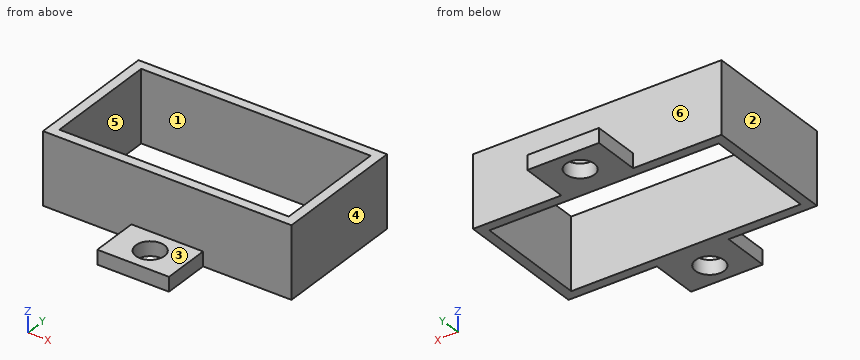
from build123d import *

# Parameters (mm, degrees)
SKETCH_1_W          = 52
SKETCH_1_H          = 28
SKETCH_1_W_2        = 48
SKETCH_1_H_2        = 24
EXTRUDE_1_DEPTH     = 15
SKETCH_2_W          = 15
SKETCH_2_H          = 3
EXTRUDE_2_DEPTH     = 10
SKETCH_3_R          = 3
CUT_EXTRUDE_1_DEPTH = 10


with BuildPart() as part:
    # 草圖1 → 填料-伸長1 (new body)
    with BuildSketch(Plane.XY):
        Rectangle(SKETCH_1_W, SKETCH_1_H)
        Rectangle(SKETCH_1_W_2, SKETCH_1_H_2, mode=Mode.SUBTRACT)
    extrude(amount=EXTRUDE_1_DEPTH)

    # 草圖2 → 填料-伸長2 (add)
    with BuildSketch(Plane(origin=(0, 14, 0), x_dir=(1, 0, 0), z_dir=(0, 1, 0))):
        with Locations((0, -1.5)):
            Rectangle(SKETCH_2_W, SKETCH_2_H)
    extrude_2 = extrude(amount=EXTRUDE_2_DEPTH)

    # 草圖3 → 除料-伸長1 (cut)
    with BuildSketch(Plane.XY.offset(3)):
        with Locations((0, 19)):
            Circle(SKETCH_3_R)
    cut_extrude_1 = extrude(amount=-CUT_EXTRUDE_1_DEPTH, mode=Mode.SUBTRACT)

    # 鏡射1: 填料-伸長2, 除料-伸長1 across plane
    add(extrude_2.mirror(Plane.ZX))
    add(cut_extrude_1.mirror(Plane.ZX), mode=Mode.SUBTRACT)


solid = part.part
Input: part model. Units: mm. Frame: model coordinates. Face numbers are marked on the shaded views. A direction names the side the tool comes from. Coordinates: 2 decimals unless noted, no trailing zeros. Loops run counter-clockwise (first coordinate to the right, second up) from the corner with the lowest first, then second, coordinate; pieces in that order, holes last. Notation, with made-up numbers: (14.5, 2.25) - (25.5, 2.25) arc R20 cw to (25.5, 39.25) - close; hole circle Ø5 at (77, 67.5). An arc over 180 degrees is marked (long way). Answer in a Markdown table with one row per item. Add a question column.
Item 1: Contact query for flat-ended pins moving along their axis: P1, Ø2, axis at x = -5.5, y = 16.5, coming from the +Z side; P2, Ø1.5, axis at y = -20, z = 1, coming from the -X side; P3, Ø0.9, axis at y = 20, z = 1, coming from the +X side; P4, Ø10, axis at x = 11.5, y = -6, coming from the +Z side. Output: stop coordinate, or through.
Item 2: Section query D-D on x = -15. Return the cut outline in (y, z).
Item 3: Section query B-B on y = -19. Return the cut outline in (x, z), then the cut area to 3 significant figures.
Item 4: Access query for the marked faces 1, 2 and 3. Directions: +Z, -Z, +X, -X, +Y, -Y. A direction counts if a zero-diameter tool reaches every point of the face in a straight line with its end or side. Return the directions, or none.
Item 5: Section query C-C on z = 4.75. Return the cut outline in (x, y), then the cut area to 3 significant figures.
Item 6: Line query: line 1 along Y through (x, z) = (0, 1.95); line 2 along Y through (x, z) = (-18, 6.5); line 3 along X through (y, z) = (-19, 1). Output: solid intervals per line, ascending. Write a range as [from, to].
Item 7: Mould query, pull axis X, two halves, no side actions, for the marked faces 4, 5 and 6. Classes: released by +X, released by -X, zero draft, split by the parting line, or undercut.
Item 8: Section query A-A on x = 0. Return the cut outline in (y, z), then the cut area to 3 significant figures.
Recorded:
| question | item | result |
|---|---|---|
| 1 | P1 | z = 3 |
| 1 | P2 | x = -7.5 |
| 1 | P3 | x = 7.5 |
| 1 | P4 | through |
| 2 | outline | (-14, 0) - (-12, 0) - (-12, 15) - (-14, 15) - close; (12, 0) - (14, 0) - (14, 15) - (12, 15) - close |
| 3 | outline | (-7.5, 0) - (-3, 0) - (-3, 3) - (-7.5, 3) - close; (3, 0) - (7.5, 0) - (7.5, 3) - (3, 3) - close |
| 3 | area | 27.0 mm^2 |
| 4 | face 1 | +Z, -Z |
| 4 | face 2 | +Z, -Z, -X, +Y, -Y |
| 4 | face 3 | +Z, +X, -X, -Y |
| 5 | outline | (-26, -14) - (26, -14) - (26, 14) - (-26, 14) - close; hole (-24, -12) - (24, -12) - (24, 12) - (-24, 12) - close |
| 5 | area | 304 mm^2 |
| 6 | line 1 | [-24, -22], [-16, -12], [12, 16], [22, 24] |
| 6 | line 2 | [-14, -12], [12, 14] |
| 6 | line 3 | [-7.5, -3], [3, 7.5] |
| 7 | face 4 | released by +X |
| 7 | face 5 | undercut |
| 7 | face 6 | zero draft |
| 8 | outline | (-24, 0) - (-22, 0) - (-22, 3) - (-24, 3) - close; (-16, 0) - (-12, 0) - (-12, 15) - (-14, 15) - (-14, 3) - (-16, 3) - close; (12, 0) - (16, 0) - (16, 3) - (14, 3) - (14, 15) - (12, 15) - close; (22, 0) - (24, 0) - (24, 3) - (22, 3) - close |
| 8 | area | 84.0 mm^2 |
